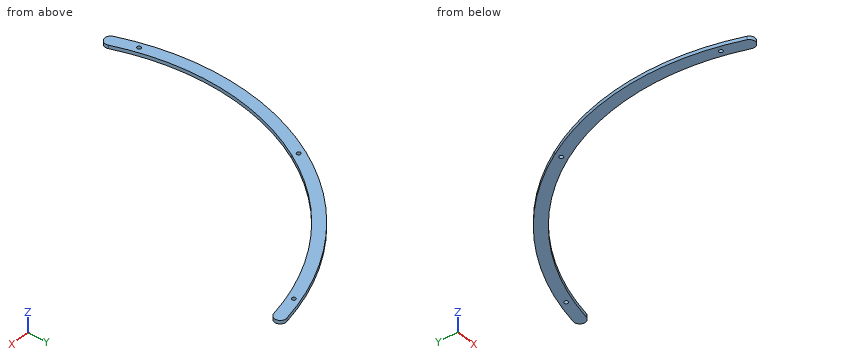
```python
from build123d import *

# Parameters (mm, degrees)
PAD014_DEPTH                        = 3
SKETCH055_R                         = 1.65
POCKET019_DEPTH                     = 364.282338
POCKET019_DEPTH_BACK                = 367.282338
BODY001003005003003_PLACEMENT_ANGLE = 60


with BuildPart() as part:
    # Sketch052 → Pad014 (new body)
    with BuildSketch(Plane.XY):
        with BuildLine():
            ThreePointArc((152.959511, 127.101705), (84.480895, 180.040089), (0, 198.875477))
            Line((0, 198.875477), (0, 208.875477))
            ThreePointArc((160.650731, 133.492724), (88.728824, 189.092995), (0, 208.875477))
            ThreePointArc((152.959511, 127.101705), (160.000631, 126.451604), (160.650731, 133.492724))
        make_face()
    pad014 = extrude(amount=PAD014_DEPTH)

    # Sketch055 → Pocket019 (cut, two sides)
    with BuildSketch(Plane.XY) as pocket019_sk:
        with Locations((143.11, 145.205847)):
            Circle(SKETCH055_R)
        with BuildLine():
            Line((0, 202.225477), (0, 205.525477))
            ThreePointArc((0, 202.225477), (1.65, 203.875477), (0, 205.525477))
        make_face()
    pocket019 = extrude(amount=-POCKET019_DEPTH, mode=Mode.SUBTRACT) + extrude(pocket019_sk.sketch, amount=POCKET019_DEPTH_BACK, mode=Mode.SUBTRACT)

    # Mirrored019: Pad014, Pocket019 across Sketch052 V_Axis
    add(pad014.mirror(Plane(origin=(0, 0, 0), x_dir=(0, 0, 1), z_dir=(1, 0, 0))))
    add(pocket019.mirror(Plane(origin=(0, 0, 0), x_dir=(0, 0, 1), z_dir=(1, 0, 0))), mode=Mode.SUBTRACT)


with BuildPart() as part_1:
    # Body001003005003003 placement: moved
    add(part.part.rotate(Axis((0, 0, 0), (0, 0, 1)), BODY001003005003003_PLACEMENT_ANGLE))


solid = part_1.part
```
Verification items for the finished model (mm, model axes). Coordinates: 2 decimals unless noted, no trailing zeros. Loops run counter-clockwise (first coordinate to the right, second up) from the corner with the lowest first, then second, coordinate; pieces in that order, holes last. Notation, with made-up numbers: (23, -20.75) - (50, -20.75) arc R25 ccw to (50, -2.75) - close; hole circle Ø5 at (-17, -11.75). An arc over 180 degrees is marked (long way). Answer as a JSON object with one key per item and string values.
(1) Scan lines: line 1 along X through (y, z) = (-2.5, 2); line 2 along X through (y, z) = (-30.5, 2.4); line 3 along Y through (x, z) = (-116.5, 1.1). Record each from-to range of solid material in increasing order.
Response:
{"line 1": "x = -208.86 to -198.86", "line 2": "x = -206.64 to -196.52", "line 3": "y = 161.18 to 173.37"}
(2) Cross-section at A-A, the plane z = 1.85. Record the boundary of the cut face in (x, y).
Response:
{"outline": "(-195.93, -72.38) arc R5 ccw to (-186.55, -68.92) arc R198.88 cw to (-172.23, 99.44) arc R198.88 cw to (-33.59, 196.02) arc R5 ccw to (-35.28, 205.87) arc R208.88 ccw to (-180.89, 104.44) arc R208.88 ccw to start; hole circle Ø3.3 at (-197.31, -51.33); hole circle Ø3.3 at (-176.56, 101.94); hole circle Ø3.3 at (-54.2, 196.54)"}
(3) Cross-section at C-C, the plane x = -116.5. Record the boundary of the cut face in (y, z).
Response:
{"outline": "(161.18, 0) - (173.37, 0) - (173.37, 3) - (161.18, 3) - close"}
(4) Cross-section at B-B, the plane y = 81. Record the boundary of the cut face in (x, z), then the cut area to 3 significant figures.
Response:
{"outline": "(-192.53, 0) - (-181.63, 0) - (-181.63, 3) - (-192.53, 3) - close", "area": "32.7 mm²"}
(5) Go/stop test with a flat-tipped pin: pin 1 Ø2 at (x, y) = (-176.56, 101.94) entering from +Z. Record where the tip stops, or that it passes through.
Response:
{"pin 1": "passes through"}
